```python
from build123d import *

# Parameters (mm, degrees)
SKETCH_1_R          = 1.5
EXTRUDE_1_DEPTH     = 1
SKETCH_3_W          = 18
SKETCH_3_H          = 14
SKETCH_3_W_2        = 20
SKETCH_3_H_2        = 15
EXTRUDE_2_DEPTH     = 15
SKETCH_4_W          = 12
SKETCH_4_H          = 5.4
SKETCH_4_W_2        = 9.6
SKETCH_4_H_2        = 1.7
CUT_EXTRUDE_1_DEPTH = 14
SKETCH_5_W          = 13
SKETCH_5_H          = 12
CUT_EXTRUDE_2_DEPTH = 14
SKETCH_2_W          = 50
SKETCH_2_H          = 5
EXTRUDE_3_DEPTH     = 5
SKETCH_7_W          = 14
SKETCH_7_H          = 1
CUT_EXTRUDE_5_DEPTH = 5


with BuildPart() as part:
    # Эскиз1 → Бобышка-Вытянуть1 (new body)
    with BuildSketch(Plane(origin=(0, 0, 0), x_dir=(1, 0, 0), z_dir=(0, 1, 0))):
        with BuildLine():
            Line((1, 0), (83, 0))
            ThreePointArc((83, 0), (83.707106781, 0.292893219), (84, 1))
            Line((84, 1), (84, 55))
            ThreePointArc((84, 55), (83.707106781, 55.707106781), (83, 56))
            Line((83, 56), (1, 56))
            ThreePointArc((1, 56), (0.292893219, 55.707106781), (0, 55))
            Line((0, 55), (0, 1))
            ThreePointArc((0, 1), (0.292893219, 0.292893219), (1, 0))
        make_face()
        with Locations(Location((3, 53, 0), (0, 0, 270))):
            Circle(SKETCH_1_R, mode=Mode.SUBTRACT)
        with Locations(Location((61, 53, 0), (0, 0, 270))):
            Circle(SKETCH_1_R, mode=Mode.SUBTRACT)
        with Locations(Location((61, 3, 0), (0, 0, 270))):
            Circle(SKETCH_1_R, mode=Mode.SUBTRACT)
        with Locations(Location((3, 3, 0), (0, 0, 270))):
            Circle(SKETCH_1_R, mode=Mode.SUBTRACT)
    extrude(amount=EXTRUDE_1_DEPTH)

    # Эскиз3 → Бобышка-Вытянуть2 (add)
    with BuildSketch(Plane(origin=(0, 1, 0), x_dir=(1, 0, 0), z_dir=(0, 1, 0))):
        with Locations((77, 28.5)):
            Rectangle(SKETCH_3_W, SKETCH_3_H)
        with Locations((76, 10)):
            Rectangle(SKETCH_3_W_2, SKETCH_3_H_2)
        with Locations((77, 46.5)):
            Rectangle(SKETCH_3_W, SKETCH_3_H)
    extrude(amount=EXTRUDE_2_DEPTH)

    # Эскиз4 → Вырез-Вытянуть1 (cut)
    # profile 1 of 4: a face of its own
    with BuildSketch(Plane(origin=(86, 0, 0), x_dir=(0, 0, -1), z_dir=(1, 0, 0))):
        with Locations((46.5, 12.8)):
            Rectangle(SKETCH_4_W, SKETCH_4_H)
        with Locations((46.5, 13.75)):
            Rectangle(SKETCH_4_W_2, SKETCH_4_H_2, mode=Mode.SUBTRACT)
    # profile 2 of 4: a face of its own
    with BuildSketch(Plane(origin=(86, 0, 0), x_dir=(0, 0, -1), z_dir=(1, 0, 0))):
        with Locations((46.5, 5.2)):
            Rectangle(SKETCH_4_W, SKETCH_4_H)
        with Locations((46.5, 6.15)):
            Rectangle(SKETCH_4_W_2, SKETCH_4_H_2, mode=Mode.SUBTRACT)
    # profile 3 of 4: a face of its own
    with BuildSketch(Plane(origin=(86, 0, 0), x_dir=(0, 0, -1), z_dir=(1, 0, 0))):
        with Locations((28.5, 5.2)):
            Rectangle(SKETCH_4_W, SKETCH_4_H)
        with Locations((28.5, 6.15)):
            Rectangle(SKETCH_4_W_2, SKETCH_4_H_2, mode=Mode.SUBTRACT)
    # profile 4 of 4: a face of its own
    with BuildSketch(Plane(origin=(86, 0, 0), x_dir=(0, 0, -1), z_dir=(1, 0, 0))):
        with Locations((28.5, 12.8)):
            Rectangle(SKETCH_4_W, SKETCH_4_H)
        with Locations((28.5, 13.75)):
            Rectangle(SKETCH_4_W_2, SKETCH_4_H_2, mode=Mode.SUBTRACT)
    extrude(amount=-CUT_EXTRUDE_1_DEPTH, mode=Mode.SUBTRACT)

    # Эскиз5 → Вырез-Вытянуть2 (cut)
    with BuildSketch(Plane(origin=(86, 0, 0), x_dir=(0, 0, -1), z_dir=(1, 0, 0))):
        with Locations((10, 8.5)):
            Rectangle(SKETCH_5_W, SKETCH_5_H)
    extrude(amount=-CUT_EXTRUDE_2_DEPTH, mode=Mode.SUBTRACT)

    # Эскиз2 → Бобышка-Вытянуть3 (add)
    with BuildSketch(Plane(origin=(0, 1, 0), x_dir=(1, 0, 0), z_dir=(0, 1, 0))):
        with Locations((32, 52.567639547)):
            Rectangle(SKETCH_2_W, SKETCH_2_H)
    extrude(amount=EXTRUDE_3_DEPTH)

    # Эскиз7 → Вырез-Вытянуть5 (cut)
    with BuildSketch(Plane(origin=(86, 0, 0), x_dir=(0, 0, -1), z_dir=(1, 0, 0))):
        with Locations((28.5, 1.5)):
            Rectangle(SKETCH_7_W, SKETCH_7_H)
        with Locations((46.5, 1.5)):
            Rectangle(SKETCH_7_W, SKETCH_7_H)
    extrude(amount=-CUT_EXTRUDE_5_DEPTH, mode=Mode.SUBTRACT)


solid = part.part
```
Design review of the part built by this model. Coordinates are the model's own, in mm. A direction names the side the tool comes from. Coordinates: 2 decimals unless noted, no trailing zeros. Loops run counter-clockwise (first coordinate to the right, second up) from the corner with the lowest first, then second, coordinate; pieces in that order, holes last.
Q1. The part is to be moulded in two halves that separate along Z. For faces 1 (the face through (32, 6, -53)), 2 (the face through (77, 8, -53.5)), 3 (the face through (72, 5, -46)), say which applies: +Z half, -Z half, draft (parallel to the pull), parting line (faces both ways), or undercut.
Reported:
face 1: draft
face 2: -Z half
face 3: undercut
Q2. We need section A-A on y = 4. State the section outline as (x, z) points, and give its area (3 significant figures).
Reported:
outline: (7, -55.07) - (57, -55.07) - (57, -50.07) - (7, -50.07) - close; (66, -17.5) - (86, -17.5) - (86, -16.5) - (72, -16.5) - (72, -3.5) - (86, -3.5) - (86, -2.5) - (66, -2.5) - close; (68, -53.5) - (86, -53.5) - (86, -52.5) - (72, -52.5) - (72, -40.5) - (86, -40.5) - (86, -39.5) - (68, -39.5) - close; (68, -35.5) - (86, -35.5) - (86, -34.5) - (72, -34.5) - (72, -22.5) - (86, -22.5) - (86, -21.5) - (68, -21.5) - close
area: 536 mm2
Q3. To check wall thickness, follow line 1 (X direction, y = 0.5, z = -53); line 2 (Y direction, x = 77, z = -14); line 3 (Y direction, x = 57, z = -40.5). State the ranges of each line that lie inside material, in increasing order.
Reported:
line 1: x = 0 to 1.5, 4.5 to 59.5, 62.5 to 84
line 2: y = 0 to 2.5, 14.5 to 16
line 3: y = 0 to 1
Q4. We need section B-B on x = 61. State the section outline as (y, z) points, and give its area (3 significant figures).
Reported:
outline: (0, -56) - (1, -56) - (1, -54.5) - (0, -54.5) - close; (0, -51.5) - (1, -51.5) - (1, -4.5) - (0, -4.5) - close; (0, -1.5) - (1, -1.5) - (1, 0) - (0, 0) - close
area: 50.0 mm2
Q5. We need section C-C on z = -46. State the section outline as (x, y) points.
Reported:
outline: (0, 0) - (84, 0) - (84, 1) - (81, 1) - (81, 2) - (86, 2) - (86, 2.5) - (72, 2.5) - (72, 5.3) - (86, 5.3) - (86, 7) - (72, 7) - (72, 7.9) - (86, 7.9) - (86, 10.1) - (72, 10.1) - (72, 12.9) - (86, 12.9) - (86, 14.6) - (72, 14.6) - (72, 15.5) - (86, 15.5) - (86, 16) - (68, 16) - (68, 1) - (0, 1) - close
Q6. For pin 1 (4 mm diameter, centred on y = 10, z = -31, fed in from -X); pin 2 (10.5 mm diameter, centred on x = 81, z = -48.5, fed in from -Y); pin 3 (0.5 mm diameter, centred on y = 0.5, z = -29, fed in from +X); pin 4 (5 mm diameter, centred on x = 38.5, z = -32.5, fed in from +Y), all flat-tipped, find the tip position at first contact; note any pin that passes through.
Reported:
pin 1: stops at x = 68
pin 2: stops at y = 0
pin 3: stops at x = 84
pin 4: stops at y = 1
Q7. We need section D-D on x = 14. State the section outline as (y, z) points, and give its area (3 significant figures).
Reported:
outline: (0, -56) - (1, -56) - (1, -55.07) - (6, -55.07) - (6, -50.07) - (1, -50.07) - (1, 0) - (0, 0) - close
area: 81.0 mm2
Q8. Tool access review of faces 4 (the face through (32, 3, -50.068)), 5 (the face through (57, 3, -53)), 6 (the face through (79, 2.5, -10)): name each direction out of +Z, -Z, +X, -X, +Y, -Y from which nothing blocks a thin tool from reaching the whole face with its end or side.
Reported:
face 4: +Z, -X, +Y
face 5: +Z, -Z, +Y
face 6: +X
